Verification items for the finished model (mm, model axes). Face numbers are marked on the shaded views. Round coordinates to 2 decimals unless told otherwise and drop trailing zeros. Loops run counter-clockwise (first coordinate to the right, second up) from the corner with the lowest first, then second, coordinate; pieces in that order, holes last.
from build123d import *

# Parameters (mm, degrees)
F0_R     = 15
F0_R_2   = 5
F1_DEPTH = 9
F2_R     = 1


with BuildPart() as f1:
    # F0 (on Front) → F1 (new body)
    with BuildSketch(Plane.XZ):
        Circle(F0_R)
        Circle(F0_R_2, mode=Mode.SUBTRACT)
    extrude(amount=F1_DEPTH)

    # F2
    f2_edges = [f1.edges().sort_by_distance(p)[0] for p in [
        (15, -4.5, 0),
        (-15, 0, 0),
        (-15, -9, 0),
        (5, -4.5, 0),
        (-5, 0, 0),
        (-5, -9, 0),
    ]]
    fillet(f2_edges, radius=F2_R)


solid = f1.part
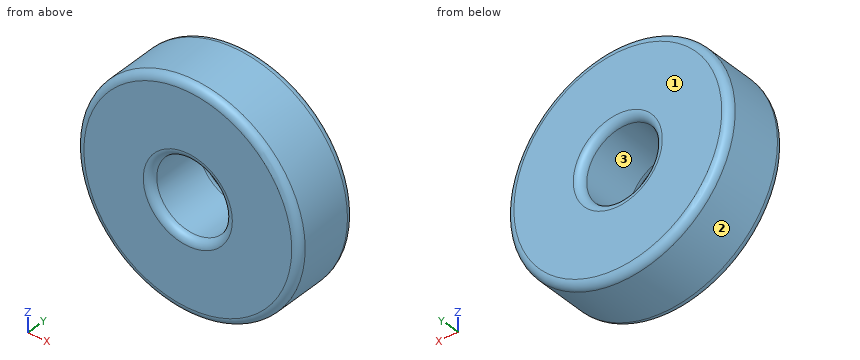
1. Section check B-B (z = 0). Enter the section's corners in (x, y), then the cut area to 3 significant figures.
2. Release check for a two-part mould opening along X. For the marked faces 1, 2 and 3 record: released by +X, released by -X, zero draft, split by the parting line, or undercut.
3. Section check C-C (y = -3). Enter the section's corners in (x, z).
4. Section check D-D (y = -8.5). Enter the section's corners in (x, z), then the cut area to 3 significant figures.
5. Section check A-A (x = 0). Enter the section's corners in (y, z).
6. Scan lines: L1, parallel to Z at x = 0, y = -3.25; L2, parallel to X at y = -7, z = -0.5; L3, parallel to X at y = -2, z = 1.75. Record each from-to range of solid material in increasing order.
7. Gauge pin test, flat ends, axial feed: P1, Ø1.5, axis at y = -4.5, z = 9, coming from the -X side; P2, Ø5, axis at x = -1.5, z = 6.5, coming from the +Y side; P3, Ø1.5, axis at x = -9, y = -2, coming from the +Z side; P4, Ø3, axis at y = -7.5, z = -5.5, coming from the +X side. Record the tip position at first contact, or that the pin passes through.
Taken from the geometry:
1. outline: (-15, -8) arc R1 ccw to (-14, -9) - (-6, -9) arc R1 ccw to (-5, -8) - (-5, -1) arc R1 ccw to (-6, 0) - (-14, 0) arc R1 ccw to (-15, -1) - close; (5, -8) arc R1 ccw to (6, -9) - (14, -9) arc R1 ccw to (15, -8) - (15, -1) arc R1 ccw to (14, 0) - (6, 0) arc R1 ccw to (5, -1) - close
1. area: 178 mm2
2. face 1: zero draft
2. face 2: split by the parting line
2. face 3: undercut
3. outline: circle Ø30 at (0, 0); hole circle Ø10 at (0, 0)
4. outline: circle Ø29.73 at (0, 0); hole circle Ø10.27 at (0, 0)
4. area: 611 mm2
5. outline: (-9, -14) arc R1 ccw to (-8, -15) - (-1, -15) arc R1 ccw to (0, -14) - (0, -6) arc R1 ccw to (-1, -5) - (-8, -5) arc R1 ccw to (-9, -6) - close; (-9, 6) arc R1 ccw to (-8, 5) - (-1, 5) arc R1 ccw to (0, 6) - (0, 14) arc R1 ccw to (-1, 15) - (-8, 15) arc R1 ccw to (-9, 14) - close
6. L1: z = -15 to -5, 5 to 15
6. L2: x = -14.99 to -4.97, 4.97 to 14.99
6. L3: x = -14.9 to -4.68, 4.68 to 14.9
7. P1: stops at x = -12.53
7. P2: stops at y = 0
7. P3: stops at z = 12.53
7. P4: stops at x = 14.46
